from build123d import *

# Parameters (mm, degrees)
ESQUISSE1_R             = 1.65
BOSS_EXTRU_1_DEPTH      = 8
ESQUISSE2_R             = 1.75
ENL_V_MAT_EXTRU_1_DEPTH = 33.57299495
CONG_1_R                = 3
ESQUISSE3_W             = 5
ESQUISSE3_H             = 7
ENL_V_MAT_EXTRU_2_DEPTH = 33.57299495


with BuildPart() as part:
    # Esquisse1 → Boss.-Extru.1 (new body)
    with BuildSketch(Plane.XY):
        Polygon((0, 0), (6, 0), (6, 6.5), (3, 6.5), (3, 24.5), (6, 24.5), (6, 31), (0, 31), align=None)
        with Locations((3, 28)):
            Circle(ESQUISSE1_R, mode=Mode.SUBTRACT)
        with Locations(Location((3, 3, 0), (0, 0, 180))):
            Circle(ESQUISSE1_R, mode=Mode.SUBTRACT)
    extrude(amount=BOSS_EXTRU_1_DEPTH)

    # Esquisse2 → Enlèv. mat.-Extru.1 (cut, through all)
    with BuildSketch(Plane.ZY):
        with Locations((4.25, 21.5)):
            Circle(ESQUISSE2_R)
        with Locations((4.25, 9.5)):
            Circle(ESQUISSE2_R)
    extrude(amount=-ENL_V_MAT_EXTRU_1_DEPTH, mode=Mode.SUBTRACT)

    # Congé1
    cong_1_edges = [part.edges().sort_by_distance(p)[0] for p in [
        (6, 0, 4),
        (0, 0, 4),
        (0, 31, 4),
        (6, 31, 4),
    ]]
    fillet(cong_1_edges, radius=CONG_1_R - 0.0001)  # a hair under: the kernel refuses the full size

    # Esquisse3 → Enlèv. mat.-Extru.2 (cut, through all)
    with BuildSketch(Plane.ZY):
        with Locations((5.5, 27.5)):
            Rectangle(ESQUISSE3_W, ESQUISSE3_H)
        with Locations((5.5, 3.5)):
            Rectangle(ESQUISSE3_W, ESQUISSE3_H)
    extrude(amount=-ENL_V_MAT_EXTRU_2_DEPTH, mode=Mode.SUBTRACT)


solid = part.part
Verification items for the finished model (mm, model axes). A direction names the side the tool comes from. Round coordinates to 2 decimals unless told otherwise and drop trailing zeros. Write each loop counter-clockwise with the first axis right and the second up, starting at its lowest first coordinate (ties: lowest second). Pieces come first, ordered by that corner, then holes.
(1) Material ranges on line 1 (Y direction, x = 3.1, z = 2.5); line 2 (Y direction, x = 4.1, z = 1.5); line 3 (Y direction, x = 2.45, z = 0.5), recorded low to high.
Returned:
line 1: y = 0 to 1.35, 4.65 to 6.5, 24.5 to 26.35, 29.65 to 31
line 2: y = 0.21 to 1.77, 4.23 to 6.5, 24.5 to 26.77, 29.23 to 30.79
line 3: y = 0.05 to 1.44, 4.56 to 26.44, 29.56 to 30.95
(2) Section check C-C (x = 5.2). Enter the section's corners in (y, z), plus the area to 3 significant figures.
Returned:
outline: (0.96, 0) - (6.5, 0) - (6.5, 3) - (0.96, 3) - close; (24.5, 0) - (30.04, 0) - (30.04, 3) - (24.5, 3) - close
area: 33.2 mm2
(3) Access from +Z, -Z, +X, -X, +Y, -Y to the whole of each face (thin tool, end or side, straight path). Record for faces 1 (the flat face through (1.6, 26.7, 3)), 2 (the cylindrical face through (5.1, 0.86, 1.52)), 3 (the flat face through (0, 16, 3)), 4 (the flat face through (1, 7, 5)), 5 (the flat face through (5, 6.5, 1)).
Returned:
face 1: +Z, +X, -X, +Y
face 2: +Z, -Z, +X, -Y
face 3: +Z, -Z, -X, +Y, -Y
face 4: +Z, +X, -X, -Y
face 5: +Z, -Z, +X
(4) Section check A-A (y = 9.5). Enter the section's corners in (x, z).
Returned:
outline: (0, 0) - (3, 0) - (3, 2.5) - (0, 2.5) - close; (0, 6) - (3, 6) - (3, 8) - (0, 8) - close
(5) Depth check by flat-ended pin: pin 1 Ø0.9 at (x, z) = (5, 2) entering from -Y; pin 2 Ø1.8 at (x, y) = (4, 28) entering from +Z; pin 3 Ø3.5 at (x, z) = (5, 1.5) entering from +Y. Enter the tip coordinate at first touch or a pass-through.
Returned:
pin 1: stops at y = 0.43
pin 2: stops at z = 3
pin 3: stops at y = 30.99
(6) Mould release check, pull along Z, two halves, no side actions. Record for faces 6 (the cylindrical face through (1.48, 10.68, 2.96)), 7 (the flat face through (1, 16, 8)), 8 (the flat face through (1, 24, 5)): pulls with the +Z half, pulls with the -Z half, needs draft (parallel to the pull), parting line crosses it, or undercut.
Returned:
face 6: undercut
face 7: pulls with the +Z half
face 8: needs draft
(7) Section check D-D (z = 1). Give the number of separate pieces and of enclosed holes in the cut face, plus the area to 3 significant figures.
Returned:
separate pieces: 1
enclosed holes: 2
area: 107 mm2
(8) Section check B-B (z = 4.25). Enter the section's corners in (x, y), plus the area to 3 significant figures.
Returned:
outline: (0, 7) - (3, 7) - (3, 7.75) - (0, 7.75) - close; (0, 11.25) - (3, 11.25) - (3, 19.75) - (0, 19.75) - close; (0, 23.25) - (3, 23.25) - (3, 24) - (0, 24) - close
area: 30.0 mm2
